Check sheet for the modelled part. Datum: model origin and axes. Units: mm. A direction names the side the tool comes from. Give positions to 0.01 mm unless a question says otherwise; leave off trailing zeros. Loops run counter-clockwise (first coordinate to the right, second up) from the corner with the lowest first, then second, coordinate; pieces in that order, holes last. Notation, with made-up numbers: (70.25, 36) - (115.25, 36) arc R31 cw to (115.25, 64) - close; hole circle Ø4 at (44.5, 70.25). An arc over 180 degrees is marked (long way). Use one line per item in the form item = value.
from build123d import *

# Parameters (mm, degrees)
SKETCH1_W               = 80
SKETCH1_H               = 50
BOSS_EXTRUDE1_DEPTH     = 5
SKETCH2_R               = 3.6
CUT_EXTRUDE1_DEPTH      = 123.886126149
SKETCH3_R               = 1.5
CUT_EXTRUDE2_DEPTH      = 123.886126149
SKETCH4_R               = 11.1
CUT_EXTRUDE3_DEPTH      = 2
SKETCH5_R               = 15
CUT_EXTRUDE4_DEPTH      = 123.886126149
SKETCH6_R               = 1.75
CUT_EXTRUDE5_DEPTH      = 123.886126149
SKETCH7_W               = 80
SKETCH7_H               = 50
BOSS_EXTRUDE2_DEPTH     = 10
FILLET1_R               = 20
CUT_EXTRUDE6_DEPTH      = 140.283882772
CUT_EXTRUDE6_DEPTH_BACK = 140.283882772
SKETCH9_R               = 1.75
SKETCH10_R              = 1.75
CUT_EXTRUDE7_DEPTH      = 140.283882772
SKETCH11_R              = 1.75
CUT_EXTRUDE8_DEPTH      = 134.120246394


with BuildPart() as part:
    # Sketch1 → Boss-Extrude1 (new body)
    with BuildSketch(Plane.XY):
        with Locations((-80, -1)):
            Rectangle(SKETCH1_W, SKETCH1_H)
    extrude(amount=BOSS_EXTRUDE1_DEPTH)

    # Sketch2 → Cut-Extrude1 (cut, through all)
    with BuildSketch(Plane.XY.offset(5)):
        with Locations((-105, -1)):
            Circle(SKETCH2_R)
    extrude(amount=-CUT_EXTRUDE1_DEPTH, mode=Mode.SUBTRACT)

    # Sketch3 → Cut-Extrude2 (cut, through all)
    with BuildSketch(Plane.XY.offset(5)):
        with Locations((-96.25, -1)):
            Circle(SKETCH3_R)
        with Locations((-113.75, -1)):
            Circle(SKETCH3_R)
    extrude(amount=-CUT_EXTRUDE2_DEPTH, mode=Mode.SUBTRACT)

    # Sketch4 → Cut-Extrude3 (cut)
    with BuildSketch(Plane.XY.offset(5)):
        with Locations((-105, -1)):
            Circle(SKETCH4_R)
    extrude(amount=-CUT_EXTRUDE3_DEPTH, mode=Mode.SUBTRACT)

    # Sketch5 → Cut-Extrude4 (cut, through all)
    with BuildSketch(Plane.XY.offset(5)):
        with Locations((-64.5, -1)):
            Circle(SKETCH5_R)
    extrude(amount=-CUT_EXTRUDE4_DEPTH, mode=Mode.SUBTRACT)

    # Sketch6 → Cut-Extrude5 (cut, through all)
    with BuildSketch(Plane.XY.offset(5)):
        with Locations((-81.117009358, 15.617009358)):
            Circle(SKETCH6_R)
        with Locations((-47.882990642, -17.617009358)):
            Circle(SKETCH6_R)
    extrude(amount=-CUT_EXTRUDE5_DEPTH, mode=Mode.SUBTRACT)

    # Sketch7 → Boss-Extrude2 (add)
    with BuildSketch(Plane.XZ.offset(26)):
        with Locations((-80, 25)):
            Rectangle(SKETCH7_W, SKETCH7_H)
    extrude(amount=BOSS_EXTRUDE2_DEPTH)

    # Fillet1
    fillet1_edges = [part.edges().sort_by_distance(p)[0] for p in [
        (-120, 24, 2.5),
        (-40, 24, 2.5),
    ]]
    fillet(fillet1_edges, radius=FILLET1_R)

    # Sketch9 → Cut-Extrude6 (cut, two sides: drawn at the far end of the back side and taken through both)
    with BuildSketch(Plane(origin=(0, -26, 0), x_dir=(1, 0, 0), z_dir=(0, 1, 0)).offset(-CUT_EXTRUDE6_DEPTH_BACK)):
        with Locations(Location((-115, -10, 0), (0, 0, 270))):
            Circle(SKETCH9_R)
        with Locations(Location((-45, -10, 0), (0, 0, 270))):
            Circle(SKETCH9_R)
        with Locations(Location((-45, -45, 0), (0, 0, 270))):
            Circle(SKETCH9_R)
        with Locations(Location((-115, -45, 0), (0, 0, 270))):
            Circle(SKETCH9_R)
        with Locations(Location((-95, -10, 0), (0, 0, 270))):
            Circle(SKETCH9_R)
        with Locations(Location((-95, -45, 0), (0, 0, 270))):
            Circle(SKETCH9_R)
        with Locations(Location((-75, -10, 0), (0, 0, 270))):
            Circle(SKETCH9_R)
        with Locations(Location((-75, -45, 0), (0, 0, 270))):
            Circle(SKETCH9_R)
    extrude(amount=CUT_EXTRUDE6_DEPTH + CUT_EXTRUDE6_DEPTH_BACK, mode=Mode.SUBTRACT)

    # Sketch10 → Cut-Extrude7 (cut, through all)
    with BuildSketch(Plane(origin=(0, -26, 0), x_dir=(1, 0, 0), z_dir=(0, 1, 0))):
        with Locations(Location((-95, -27.5, 0), (0, 0, 270))):
            Circle(SKETCH10_R)
        with Locations(Location((-75, -27.5, 0), (0, 0, 270))):
            Circle(SKETCH10_R)
    extrude(amount=-CUT_EXTRUDE7_DEPTH, mode=Mode.SUBTRACT)

    # Sketch11 → Cut-Extrude8 (cut, through all)
    with BuildSketch(Plane.XY.offset(5)):
        with Locations((-89.75, -17.617009358)):
            Circle(SKETCH11_R)
    extrude(amount=-CUT_EXTRUDE8_DEPTH, mode=Mode.SUBTRACT)


solid = part.part
Item 1: Section check D-D on y = -24. Record the boundary of the cut face in (x, z).
Answer block:
outline = (-120, 0) - (-40, 0) - (-40, 5) - (-120, 5) - close
Item 2: Thickness scan on L1, parallel to Z at x = -75, y = -32.75; L2, parallel to Z at x = -45, y = -29; L3, parallel to X at y = -28, z = 10. Record the ranges inside material, lowest first.
Answer block:
L1 = 0 to 8.25, 11.75 to 25.75, 29.25 to 43.25, 46.75 to 50
L2 = 0 to 8.25, 11.75 to 43.25, 46.75 to 50
L3 = -120 to -116.75, -113.25 to -96.75, -93.25 to -76.75, -73.25 to -46.75, -43.25 to -40
Item 3: Section check B-B on z = 45. Record the boundary of the cut face in (x, y), then the cut area to 3 significant figures.
Answer block:
outline = (-120, -36) - (-116.75, -36) - (-116.75, -26) - (-120, -26) - close; (-113.25, -36) - (-96.75, -36) - (-96.75, -26) - (-113.25, -26) - close; (-93.25, -36) - (-76.75, -36) - (-76.75, -26) - (-93.25, -26) - close; (-73.25, -36) - (-46.75, -36) - (-46.75, -26) - (-73.25, -26) - close; (-43.25, -36) - (-40, -36) - (-40, -26) - (-43.25, -26) - close
area = 660 mm2
Item 4: Section check C-C on y = 7.5. Record the boundary of the cut face in (x, z), then the cut area to 3 significant figures.
Answer block:
outline = (-119.69, 0) - (-76.86, 0) - (-76.86, 5) - (-97.86, 5) - (-97.86, 3) - (-112.14, 3) - (-112.14, 5) - (-119.69, 5) - close; (-52.14, 0) - (-40.31, 0) - (-40.31, 5) - (-52.14, 5) - close
area = 245 mm2
Item 5: Mould release check, pull along Y, two halves, no side actions. Record for faces 3 (the face through (-80, 24, 2)), 4 (the face through (-40, -26.3, 19.3)), 5 (the face through (-94.746, -5.251, 4.014)), 6 (the face through (-94.82, -0.55, 1.52)): released by +Y, released by -Y, zero draft, split by the parting line, or undercut.
Answer block:
face_3 = released by +Y
face_4 = zero draft
face_5 = undercut
face_6 = undercut
Item 6: Section check A-A on x = -64.5. Record the boundary of the cut face in (y, z).
Answer block:
outline = (-36, 0) - (-16, 0) - (-16, 5) - (-26, 5) - (-26, 50) - (-36, 50) - close; (14, 0) - (24, 0) - (24, 5) - (14, 5) - close
Item 7: Access from +Z, -Z, +X, -X, +Y, -Y to the whole of each face (thin tool, end or side, straight path). Record for faces 1 (the face through (-75.67, -31.07, 46.617)), 2 (the face through (-81, -1, 5)).
Answer block:
face_1 = +Y, -Y
face_2 = +Z, +X, -X, +Y
Item 8: Gauge pin test, flat ends, axial feed: P1, Ø12, axis at y = -18, z = 43.5, coming from the -X side; P2, Ø5.5, axis at x = -95, z = 10, coming from the +Y side; P3, Ø2, axis at x = -79.5, y = -13, coming from the +Z side. Record the tip position at first contact, or that the pin passes through.
Answer block:
P1 = through
P2 = -26
P3 = 5
